Geometry: final body of the model. Coordinates: model frame, mm. A direction names the side the tool comes from. Give positions to 0.01 mm unless a question says otherwise; leave off trailing zeros. Write each loop counter-clockwise with the first axis right and the second up, starting at its lowest first coordinate (ties: lowest second). Pieces come first, ordered by that corner, then holes. Notation, with made-up numbers: (-35, 89.25) - (-26, 89.25) arc R13 ccw to (-26, 106.25) - close; hole circle Ø1 at (83.25, -31.5). An arc over 180 degrees is marked (long way). Use CSV: the item, a comma, the result in double quotes. Start each with the question number.
(1) Reachability of faces 1 (the flat face through (169, 116, 15)), 2 (the flat face through (276, 122, 10)), 3 (the flat face through (221, 221, 4)) from +Z, -Z, +X, -X, +Y, -Y: full face, straight path, thin tool, end or side. Return the list, or none.
(2) Line query: probe 1 along X at (y, z) = (161, 10.5); probe 2 along X at (y, z) = (225, 13); probe 3 along Y at (x, z) = (5, 11.25). Output: solid intervals per line, ascending. Write a range as [from, to].
(3) Draft query along Z for faces 4 (the flat face through (56, 122, 10)), 5 (the flat face through (171.7, 123.7, 8)), 6 (the flat face through (168, 0, 7)). Return one class per face: released by +Z, released by -Z, zero draft, split by the parting line, or undercut.
(4) First-contact query: pin 1 Ø1.6 at (x, y) = (158, 225) entering from +Z. Flat tip, straight axial feed; report the tip coordinate or a pass-through.
(5) Section B-B on y = 94.5. Count the separate pieces of the cut face and the enclosed holes in it, and give its area (3 significant figures).
(6) Section A-A on x = 152.5. Output: boundary loops of the cut face in (y, z).
from build123d import *

# Parameters (mm, degrees)
CYLINDER050_R     = 1.3
CYLINDER050_DEPTH = 146
CYLINDER049_R     = 1.3
CYLINDER049_DEPTH = 146
CYLINDER042_R     = 1.3
CYLINDER042_DEPTH = 146
CYLINDER041_R     = 1.3
CYLINDER041_DEPTH = 146
CYLINDER038_R     = 1.3
CYLINDER038_DEPTH = 146
CYLINDER037_R     = 1.3
CYLINDER037_DEPTH = 146
CYLINDER035_R     = 1.3
CYLINDER035_DEPTH = 146
CYLINDER033_R     = 1.3
CYLINDER033_DEPTH = 146
CYLINDER031_R     = 1.3
CYLINDER031_DEPTH = 146
CYLINDER029_R     = 1.3
CYLINDER029_DEPTH = 146
CYLINDER016_R     = 1.3
CYLINDER016_DEPTH = 146
CYLINDER015_R     = 1.3
CYLINDER015_DEPTH = 146
CYLINDER006_R     = 1.3
CYLINDER006_DEPTH = 146
CYLINDER007_R     = 1.3
CYLINDER007_DEPTH = 146
CYLINDER003_R     = 1.3
CYLINDER003_DEPTH = 146
CYLINDER005_R     = 1.3
CYLINDER005_DEPTH = 146
BOX021_W          = 92
BOX021_H          = 92
BOX021_DEPTH      = 24
BOX020_W          = 92
BOX020_H          = 92
BOX020_DEPTH      = 24
BOX019_W          = 92
BOX019_H          = 92
BOX019_DEPTH      = 24
BOX018_W          = 92
BOX018_H          = 92
BOX018_DEPTH      = 24
BOX017_W          = 92
BOX017_H          = 92
BOX017_DEPTH      = 24
BOX013_W          = 92
BOX013_H          = 92
BOX013_DEPTH      = 24
BOX004_W          = 320
BOX004_H          = 210
BOX004_DEPTH      = 2
BOX015_W          = 335
BOX015_H          = 220
BOX015_DEPTH      = 4
BOX012_W          = 10
BOX012_H          = 210
BOX012_DEPTH      = 7
BOX006_W          = 340
BOX006_H          = 10
BOX006_DEPTH      = 7
BOX003_W          = 10
BOX003_H          = 210
BOX003_DEPTH      = 15
BOX002_W          = 10
BOX002_H          = 210
BOX002_DEPTH      = 15
BOX001_W          = 340
BOX001_H          = 10
BOX001_DEPTH      = 15
BOX_W             = 340
BOX_H             = 10
BOX_DEPTH         = 15
BOX011_W          = 10
BOX011_H          = 210
BOX011_DEPTH      = 7


with BuildPart() as cilindro050:
    # Cylinder050 → Cylinder050 (new body)
    with BuildSketch(Plane(origin=(5, 103, 8), x_dir=(1, 0, 0), z_dir=(0, 0, 1))):
        Circle(CYLINDER050_R)
    extrude(amount=CYLINDER050_DEPTH)


with BuildPart() as cilindro049:
    # Cylinder049 → Cylinder049 (new body)
    with BuildSketch(Plane(origin=(5, 127, 8), x_dir=(1, 0, 0), z_dir=(0, 0, 1))):
        Circle(CYLINDER049_R)
    extrude(amount=CYLINDER049_DEPTH)


with BuildPart() as cilindro042:
    # Cylinder042 → Cylinder042 (new body)
    with BuildSketch(Plane(origin=(5, 213, 8), x_dir=(1, 0, 0), z_dir=(0, 0, 1))):
        Circle(CYLINDER042_R)
    extrude(amount=CYLINDER042_DEPTH)


with BuildPart() as cilindro041:
    # Cylinder041 → Cylinder041 (new body)
    with BuildSketch(Plane(origin=(17, 225, 8), x_dir=(1, 0, 0), z_dir=(0, 0, 1))):
        Circle(CYLINDER041_R)
    extrude(amount=CYLINDER041_DEPTH)


with BuildPart() as cilindro038:
    # Cylinder038 → Cylinder038 (new body)
    with BuildSketch(Plane(origin=(158, 225, 8), x_dir=(1, 0, 0), z_dir=(0, 0, 1))):
        Circle(CYLINDER038_R)
    extrude(amount=CYLINDER038_DEPTH)


with BuildPart() as cilindro037:
    # Cylinder037 → Cylinder037 (new body)
    with BuildSketch(Plane(origin=(182, 225, 8), x_dir=(1, 0, 0), z_dir=(0, 0, 1))):
        Circle(CYLINDER037_R)
    extrude(amount=CYLINDER037_DEPTH)


with BuildPart() as cilindro035:
    # Cylinder035 → Cylinder035 (new body)
    with BuildSketch(Plane(origin=(323, 225, 8), x_dir=(1, 0, 0), z_dir=(0, 0, 1))):
        Circle(CYLINDER035_R)
    extrude(amount=CYLINDER035_DEPTH)


with BuildPart() as cilindro033:
    # Cylinder033 → Cylinder033 (new body)
    with BuildSketch(Plane(origin=(335, 213, 8), x_dir=(1, 0, 0), z_dir=(0, 0, 1))):
        Circle(CYLINDER033_R)
    extrude(amount=CYLINDER033_DEPTH)


with BuildPart() as cilindro031:
    # Cylinder031 → Cylinder031 (new body)
    with BuildSketch(Plane(origin=(335, 127, 8), x_dir=(1, 0, 0), z_dir=(0, 0, 1))):
        Circle(CYLINDER031_R)
    extrude(amount=CYLINDER031_DEPTH)


with BuildPart() as cilindro029:
    # Cylinder029 → Cylinder029 (new body)
    with BuildSketch(Plane(origin=(335, 103, 8), x_dir=(1, 0, 0), z_dir=(0, 0, 1))):
        Circle(CYLINDER029_R)
    extrude(amount=CYLINDER029_DEPTH)


with BuildPart() as cilindro016:
    # Cylinder016 → Cylinder016 (new body)
    with BuildSketch(Plane(origin=(335, 17, 8), x_dir=(1, 0, 0), z_dir=(0, 0, 1))):
        Circle(CYLINDER016_R)
    extrude(amount=CYLINDER016_DEPTH)


with BuildPart() as cilindro015:
    # Cylinder015 → Cylinder015 (new body)
    with BuildSketch(Plane(origin=(323, 5, 8), x_dir=(1, 0, 0), z_dir=(0, 0, 1))):
        Circle(CYLINDER015_R)
    extrude(amount=CYLINDER015_DEPTH)


with BuildPart() as cilindro006:
    # Cylinder006 → Cylinder006 (new body)
    with BuildSketch(Plane(origin=(182, 5, 8), x_dir=(1, 0, 0), z_dir=(0, 0, 1))):
        Circle(CYLINDER006_R)
    extrude(amount=CYLINDER006_DEPTH)


with BuildPart() as cilindro007:
    # Cylinder007 → Cylinder007 (new body)
    with BuildSketch(Plane(origin=(158, 5, 8), x_dir=(1, 0, 0), z_dir=(0, 0, 1))):
        Circle(CYLINDER007_R)
    extrude(amount=CYLINDER007_DEPTH)


with BuildPart() as cilindro003:
    # Cylinder003 → Cylinder003 (new body)
    with BuildSketch(Plane(origin=(17, 5, 8), x_dir=(1, 0, 0), z_dir=(0, 0, 1))):
        Circle(CYLINDER003_R)
    extrude(amount=CYLINDER003_DEPTH)


with BuildPart() as cilindro005:
    # Cylinder005 → Cylinder005 (new body)
    with BuildSketch(Plane(origin=(5, 17, 8), x_dir=(1, 0, 0), z_dir=(0, 0, 1))):
        Circle(CYLINDER005_R)
    extrude(amount=CYLINDER005_DEPTH)


with BuildPart() as obj1:
    # Box021 → Box021 (new body)
    with BuildSketch(Plane(origin=(14, 124, 0), x_dir=(1, 0, 0), z_dir=(0, 0, 1))):
        with Locations((46, 46)):
            Rectangle(BOX021_W, BOX021_H)
    extrude(amount=BOX021_DEPTH)


with BuildPart() as obj2:
    # Box020 → Box020 (new body)
    with BuildSketch(Plane(origin=(124, 124, 0), x_dir=(1, 0, 0), z_dir=(0, 0, 1))):
        with Locations((46, 46)):
            Rectangle(BOX020_W, BOX020_H)
    extrude(amount=BOX020_DEPTH)


with BuildPart() as obj3:
    # Box019 → Box019 (new body)
    with BuildSketch(Plane(origin=(234, 124, 0), x_dir=(1, 0, 0), z_dir=(0, 0, 1))):
        with Locations((46, 46)):
            Rectangle(BOX019_W, BOX019_H)
    extrude(amount=BOX019_DEPTH)


with BuildPart() as obj4:
    # Box018 → Box018 (new body)
    with BuildSketch(Plane(origin=(234, 15, 0), x_dir=(1, 0, 0), z_dir=(0, 0, 1))):
        with Locations((46, 46)):
            Rectangle(BOX018_W, BOX018_H)
    extrude(amount=BOX018_DEPTH)


with BuildPart() as obj5:
    # Box017 → Box017 (new body)
    with BuildSketch(Plane(origin=(124, 15, 0), x_dir=(1, 0, 0), z_dir=(0, 0, 1))):
        with Locations((46, 46)):
            Rectangle(BOX017_W, BOX017_H)
    extrude(amount=BOX017_DEPTH)


with BuildPart() as obj6:
    # Box013 → Box013 (new body)
    with BuildSketch(Plane(origin=(14, 14, 0), x_dir=(1, 0, 0), z_dir=(0, 0, 1))):
        with Locations((46, 46)):
            Rectangle(BOX013_W, BOX013_H)
    extrude(amount=BOX013_DEPTH)


with BuildPart() as obj7:
    # Box004 → Box004 (new body)
    with BuildSketch(Plane(origin=(10, 10, 8), x_dir=(1, 0, 0), z_dir=(0, 0, 1))):
        with Locations((160, 105)):
            Rectangle(BOX004_W, BOX004_H)
    extrude(amount=BOX004_DEPTH)


with BuildPart() as obj8:
    # Box015 → Box015 (new body)
    with BuildSketch(Plane(origin=(5, 5, 4), x_dir=(1, 0, 0), z_dir=(0, 0, 1))):
        with Locations((167.5, 110)):
            Rectangle(BOX015_W, BOX015_H)
    extrude(amount=BOX015_DEPTH)


with BuildPart() as obj9:
    # Box012 → Box012 (new body)
    with BuildSketch(Plane(origin=(220, 10, 8), x_dir=(1, 0, 0), z_dir=(0, 0, 1))):
        with Locations((5, 105)):
            Rectangle(BOX012_W, BOX012_H)
    extrude(amount=BOX012_DEPTH)


with BuildPart() as base003:
    # Box006 → Box006 (new body)
    with BuildSketch(Plane(origin=(0, 110, 8), x_dir=(1, 0, 0), z_dir=(0, 0, 1))):
        with Locations((170, 5)):
            Rectangle(BOX006_W, BOX006_H)
    extrude(amount=BOX006_DEPTH)


with BuildPart() as obj10:
    # Box003 → Box003 (new body)
    with BuildSketch(Plane(origin=(330, 10, 0), x_dir=(1, 0, 0), z_dir=(0, 0, 1))):
        with Locations((5, 105)):
            Rectangle(BOX003_W, BOX003_H)
    extrude(amount=BOX003_DEPTH)


with BuildPart() as obj11:
    # Box002 → Box002 (new body)
    with BuildSketch(Plane(origin=(0, 10, 0), x_dir=(1, 0, 0), z_dir=(0, 0, 1))):
        with Locations((5, 105)):
            Rectangle(BOX002_W, BOX002_H)
    extrude(amount=BOX002_DEPTH)


with BuildPart() as base2:
    # Box001 → Box001 (new body)
    with BuildSketch(Plane(origin=(0, 220, 0), x_dir=(1, 0, 0), z_dir=(0, 0, 1))):
        with Locations((170, 5)):
            Rectangle(BOX001_W, BOX001_H)
    extrude(amount=BOX001_DEPTH)


with BuildPart() as base1:
    # Box → Box (new body)
    with BuildSketch(Plane.XY):
        with Locations((170, 5)):
            Rectangle(BOX_W, BOX_H)
    extrude(amount=BOX_DEPTH)


with BuildPart() as cut065:
    # Box011 → Box011 (new body)
    with BuildSketch(Plane(origin=(110, 10, 8), x_dir=(1, 0, 0), z_dir=(0, 0, 1))):
        with Locations((5, 105)):
            Rectangle(BOX011_W, BOX011_H)
    extrude(amount=BOX011_DEPTH)

    # Fusion: union obj9, base003, obj10, obj11, base2, base1
    add(obj9.part)
    add(base003.part)
    add(obj10.part)
    add(obj11.part)
    add(base2.part)
    add(base1.part)

    # Cut: cut obj8
    add(obj8.part, mode=Mode.SUBTRACT)

    # Fusion001: union obj7
    add(obj7.part)

    # Cut001: cut obj6
    add(obj6.part, mode=Mode.SUBTRACT)

    # Cut002: cut obj5
    add(obj5.part, mode=Mode.SUBTRACT)

    # Cut003: cut obj4
    add(obj4.part, mode=Mode.SUBTRACT)

    # Cut004: cut obj3
    add(obj3.part, mode=Mode.SUBTRACT)

    # Cut005: cut obj2
    add(obj2.part, mode=Mode.SUBTRACT)

    # Cut006: cut obj1
    add(obj1.part, mode=Mode.SUBTRACT)

    # Cut019: cut Cilindro005
    add(cilindro005.part, mode=Mode.SUBTRACT)

    # Cut020: cut Cilindro003
    add(cilindro003.part, mode=Mode.SUBTRACT)

    # Cut021: cut Cilindro007
    add(cilindro007.part, mode=Mode.SUBTRACT)

    # Cut024: cut Cilindro006
    add(cilindro006.part, mode=Mode.SUBTRACT)

    # Cut030: cut Cilindro015
    add(cilindro015.part, mode=Mode.SUBTRACT)

    # Cut031: cut Cilindro016
    add(cilindro016.part, mode=Mode.SUBTRACT)

    # Cut044: cut Cilindro029
    add(cilindro029.part, mode=Mode.SUBTRACT)

    # Cut046: cut Cilindro031
    add(cilindro031.part, mode=Mode.SUBTRACT)

    # Cut048: cut Cilindro033
    add(cilindro033.part, mode=Mode.SUBTRACT)

    # Cut050: cut Cilindro035
    add(cilindro035.part, mode=Mode.SUBTRACT)

    # Cut052: cut Cilindro037
    add(cilindro037.part, mode=Mode.SUBTRACT)

    # Cut053: cut Cilindro038
    add(cilindro038.part, mode=Mode.SUBTRACT)

    # Cut056: cut Cilindro041
    add(cilindro041.part, mode=Mode.SUBTRACT)

    # Cut057: cut Cilindro042
    add(cilindro042.part, mode=Mode.SUBTRACT)

    # Cut064: cut Cilindro049
    add(cilindro049.part, mode=Mode.SUBTRACT)

    # Cut065: cut Cilindro050
    add(cilindro050.part, mode=Mode.SUBTRACT)


solid = cut065.part
Check values:
1,face 1,"+Z, +X, -X, +Y, -Y"
1,face 2,"+Z"
1,face 3,"+X"
2,probe 1,"x = [0, 10], [110, 120], [220, 230], [330, 340]"
2,probe 2,"x = [0, 15.7], [18.3, 156.7], [159.3, 180.7], [183.3, 321.7], [324.3, 340]"
2,probe 3,"y = [0, 15.7], [18.3, 101.7], [104.3, 125.7], [128.3, 211.7], [214.3, 230]"
3,face 4,"released by +Z"
3,face 5,"undercut"
3,face 6,"zero draft"
4,pin 1,"stops at z = 8"
5,separate pieces,"5"
5,enclosed holes,"0"
5,area,"428 mm²"
6,outline,"(0, 0) - (10, 0) - (10, 4) - (5, 4) - (5, 8) - (15, 8) - (15, 10) - (10, 10) - (10, 15) - (0, 15) - close; (107, 8) - (124, 8) - (124, 10) - (120, 10) - (120, 15) - (110, 15) - (110, 10) - (107, 10) - close; (216, 8) - (225, 8) - (225, 4) - (220, 4) - (220, 0) - (230, 0) - (230, 15) - (220, 15) - (220, 10) - (216, 10) - close"
